```python
from build123d import *

# Parameters (mm, degrees)
SKETCH1_W                       = 50
SKETCH1_H                       = 60
SKETCH1_R                       = 20
BOSS_EXTRUDE1_DEPTH             = 25
CHAMFER1_SIZE                   = 2.5
F_1_4_20_TAPPED_HOLE1_REACH     = 68.191
F_1_4_20_TAPPED_HOLE1_BORE_R    = 2.5527
F_1_4_0_25_DIAMETER_HOLE1_D     = 6.35
F_1_4_0_25_DIAMETER_HOLE1_DEPTH = 10
F_1_4_0_25_DIAMETER_HOLE1_TIP   = 1.907732465


with BuildPart() as part:
    # Sketch1 → Boss-Extrude1 (new body)
    with BuildSketch(Plane(origin=(0, 0, 0), x_dir=(0, 0, -1), z_dir=(1, 0, 0))):
        with Locations((-0.046631749, 12.797960187)):
            Rectangle(SKETCH1_W, SKETCH1_H)
        with Locations((-0.046631749, 15.817960187)):
            Circle(SKETCH1_R, mode=Mode.SUBTRACT)
        with BuildLine():
            ThreePointArc((15.41920449, 3.136954335), (17.273876327, 5.817960187), (18.668359584, 8.764656039))
            ThreePointArc((18.668359584, 8.764656039), (17.346806711, 9.077144311), (16.012598617, 8.824083694))
            ThreePointArc((16.012598617, 8.824083694), (15.118822775, 8.264047714), (14.450633556, 7.447960267))
            ThreePointArc((14.450633556, 7.447960267), (14.077975631, 6.461247636), (14.039858148, 5.407196971))
            ThreePointArc((14.039858148, 5.407196971), (14.487805271, 4.125208558), (15.41920449, 3.136954335))
        make_face()
        with BuildLine():
            ThreePointArc((-16.105862115, 8.824083694), (-17.440070209, 9.077144311), (-18.761623082, 8.764656039))
            ThreePointArc((-18.761623082, 8.764656039), (-17.367139825, 5.817960187), (-15.512467988, 3.136954335))
            ThreePointArc((-15.512467988, 3.136954335), (-14.581068769, 4.125208558), (-14.133121646, 5.407196971))
            ThreePointArc((-14.133121646, 5.407196971), (-14.17123911, 6.461247542), (-14.543896959, 7.447960101))
            ThreePointArc((-14.543896959, 7.447960101), (-15.212086202, 8.264047651), (-16.105862115, 8.824083694))
        make_face()
        with BuildLine():
            ThreePointArc((18.668359584, 8.764656039), (19.462739812, 11.415185915), (19.883693667, 14.149988727))
            ThreePointArc((19.883693667, 14.149988727), (18.69234004, 10.946124329), (16.012598617, 8.824083694))
            ThreePointArc((16.012598617, 8.824083694), (17.346806711, 9.077144311), (18.668359584, 8.764656039))
        make_face()
        with BuildLine():
            ThreePointArc((11.363036616, -0.6082222), (13.520968398, 1.123735939), (15.41920449, 3.136954335))
            ThreePointArc((15.41920449, 3.136954335), (14.487805271, 4.125208558), (14.039858148, 5.407196971))
            ThreePointArc((14.039858148, 5.407196971), (13.541987762, 2.025452506), (11.363036616, -0.6082222))
        make_face()
        with BuildLine():
            ThreePointArc((-16.105862115, 8.824083694), (-18.785603538, 10.946124329), (-19.976957166, 14.149988727))
            ThreePointArc((-19.976957166, 14.149988727), (-19.55600331, 11.415185915), (-18.761623082, 8.764656039))
            ThreePointArc((-18.761623082, 8.764656039), (-17.440070209, 9.077144311), (-16.105862115, 8.824083694))
        make_face()
        with BuildLine():
            ThreePointArc((-14.133121646, 5.407196971), (-14.581068769, 4.125208558), (-15.512467988, 3.136954335))
            ThreePointArc((-15.512467988, 3.136954335), (-13.614231896, 1.123735939), (-11.456300114, -0.6082222))
            ThreePointArc((-11.456300114, -0.6082222), (-13.63525126, 2.025452506), (-14.133121646, 5.407196971))
        make_face()
    extrude(amount=BOSS_EXTRUDE1_DEPTH)

    # Chamfer1
    chamfer1_edges = [part.edges().sort_by_distance(p)[0] for p in [
        (0, 12.797960187, -24.953368251),
        (0, 12.797960187, 25.046631749),
        (0, 42.797960187, 0.046631749),
        (12.5, 42.797960187, -24.953368251),
        (12.5, 42.797960187, 25.046631749),
        (25, 42.797960187, 0.046631749),
        (25, 12.797960187, 25.046631749),
        (25, 12.797960187, -24.953368251),
    ]]
    chamfer(chamfer1_edges, length=CHAMFER1_SIZE)

    # 1/4-20 Tapped Hole1 bore (on position points) → 1/4-20 Tapped Hole1 (cut, up to next)
    with BuildSketch(Plane(origin=(12.5, 42.797960187, 0.046631749), x_dir=(0, 0, 1), z_dir=(0, 1, 0)), mode=Mode.PRIVATE) as f_1_4_20_tapped_hole1_sk1:
        Circle(F_1_4_20_TAPPED_HOLE1_BORE_R)
    f_1_4_20_tapped_hole1_tool1 = extrude(f_1_4_20_tapped_hole1_sk1.sketch, amount=-F_1_4_20_TAPPED_HOLE1_REACH, mode=Mode.PRIVATE) & part.part
    add(f_1_4_20_tapped_hole1_tool1.solids().sort_by_distance((12.5, 42.79796, 0.046632))[0], mode=Mode.SUBTRACT)

    # 1/4 (0.25) Diameter Hole1
    with Locations(Plane(origin=(12.5, -17.202039813, 15.046631749), x_dir=(0, 0, -1), z_dir=(0, -1, 0))):
        with Locations((0, 0), (30, 0)):
            Hole(F_1_4_0_25_DIAMETER_HOLE1_D / 2, depth=F_1_4_0_25_DIAMETER_HOLE1_DEPTH)
            with Locations((0, 0, -(F_1_4_0_25_DIAMETER_HOLE1_DEPTH + F_1_4_0_25_DIAMETER_HOLE1_TIP / 2))):  # 118° drill point
                Cone(0, F_1_4_0_25_DIAMETER_HOLE1_D / 2, F_1_4_0_25_DIAMETER_HOLE1_TIP, mode=Mode.SUBTRACT)


solid = part.part
```
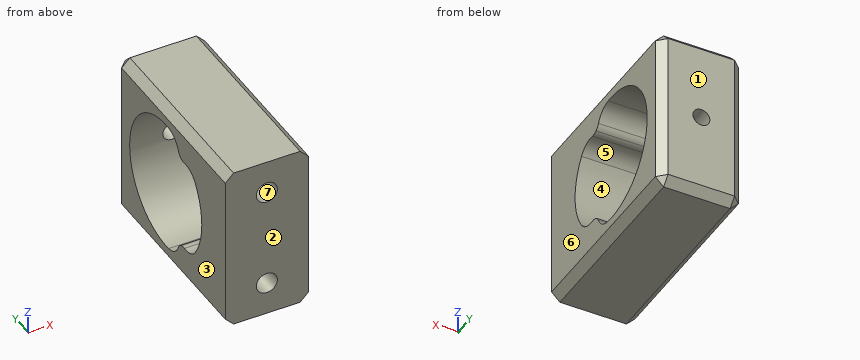
Read the model definition and answer for the solid it produces. Units are mm, in the model's axes. Face numbers are marked on the shaded views. A direction names the side the tool comes from. Round coordinates to 2 decimals unless told otherwise and drop trailing zeros. Write each loop counter-clockwise with the first axis right and the second up, starting at its lowest first coordinate (ties: lowest second). Pieces come first, ordered by that corner, then holes. Notation, with made-up numbers: (-20, 30) -> (7, 30) arc R9 cw to (7, 39) -> close; hole circle Ø10 at (-12, 55.5). An arc over 180 degrees is marked (long way). Answer in a Markdown table with one row per item. Add a question column.
1) Consider line 1 (Z direction, x = 8.5, y = 5); line 2 (Y direction, x = 3.5, z = -5.5); line 3 (Y direction, x = 11.25, z = -17). Determine where each line is inside the solid, lowest interval first.
2) Find section A-A, the plane y = 38. Determine the outline of the cut face in (x, z), and give its area (3 significant figures).
3) Find section D-D, the plane x = 20. Determine the outline of the cut face in (y, z), and give its area (3 significant figures).
4) Find section B-B, the plane z = 19. Determine the outline of the cut face in (x, y), and give its area (3 significant figures).
5) Determine the mould class of the marked faces 1, 2, 3 and 4 for opening direction Y: pulls with the +Y half, pulls with the -Y half, needs draft (parallel to the pull), parting line crosses it, or undercut.
6) Given P1, Ø5.5, axis at x = 12.5, z = 15.05, coming from the -Y side; P2, Ø4, axis at x = 12.5, z = -14.95, coming from the -Y side, each flat-ended and moving along its own axis, determine where each tip first touches the part or whether it passes through.
7) Find section C-C, the plane z = 0. Determine the outline of the cut face in (x, y), and give its area (3 significant figures).
8) Which of the six approach directions +Z, -Z, +X, -X, +Y, -Y give full straight-line access (tool end or side, diameter ignored) to the marked faces 5, 6 and 7?
Findings below:
| question | item | result |
|---|---|---|
| 1 | line 1 | -24.95 to -14.08, 14.17 to 25.05 |
| 1 | line 2 | -17.2 to -3.4, 35.03 to 42.8 |
| 1 | line 3 | -6.74 to 9.34, 26.28 to 42.8 |
| 2 | outline | (0, -22.45) -> (2.5, -24.95) -> (22.5, -24.95) -> (25, -22.45) -> (25, 22.55) -> (22.5, 25.05) -> (2.5, 25.05) -> (0, 22.55) -> close; hole circle Ø5.11 at (12.5, 0.05) |
| 2 | area | 1,220 mm² |
| 3 | outline | (-17.2, -24.95) -> (40.3, -24.95) -> (42.8, -22.45) -> (42.8, 22.55) -> (40.3, 25.05) -> (-17.2, 25.05) -> close; hole (-0.61, -11.36) arc R6.35 ccw to (5.41, -14.04) arc R3.26 cw to (8.82, -16.01) arc R6.35 ccw to (14.15, -19.88) arc R20 ccw (long way) to (14.15, 19.98) arc R6.35 ccw to (8.82, 16.11) arc R3.26 cw to (5.41, 14.13) arc R6.35 ccw to (-0.61, 11.46) arc R20 ccw to start |
| 3 | area | 1,780 mm² |
| 4 | outline | (0, -17.2) -> (25, -17.2) -> (25, 11.26) -> (0, 11.26) -> close; (0, 22.2) -> (25, 22.2) -> (25, 40.3) -> (22.5, 42.8) -> (2.5, 42.8) -> (0, 40.3) -> close |
| 4 | area | 1,220 mm² |
| 5 | face 1 | pulls with the +Y half |
| 5 | face 2 | pulls with the -Y half |
| 5 | face 3 | needs draft |
| 5 | face 4 | undercut |
| 6 | P1 | y = -6.95 |
| 6 | P2 | y = -6.5 |
| 7 | outline | (0, -17.2) -> (25, -17.2) -> (25, -4.18) -> (0, -4.18) -> close; (0, 35.82) -> (9.95, 35.82) -> (9.95, 42.8) -> (2.5, 42.8) -> (0, 40.3) -> close; (15.05, 35.82) -> (25, 35.82) -> (25, 40.3) -> (22.5, 42.8) -> (15.05, 42.8) -> close |
| 7 | area | 458 mm² |
| 8 | face 5 | +X, -X |
| 8 | face 6 | +Z, -Z, +X, +Y, -Y |
| 8 | face 7 | -Y |
